Verification items for the finished model (mm, model axes). Round coordinates to 2 decimals unless told otherwise and drop trailing zeros. Order: outer loops, then holes, each group sorted by start corner. A loop starts at its lowest first (then second) coordinate and runs counter-clockwise, first axis right, second up.
```python
from build123d import *

# Parameters (mm, degrees)
BOSS_EXTRUDE1_DEPTH = 5
CUT_EXTRUDE1_DEPTH  = 1.5
CUT_EXTRUDE2_DEPTH  = 117.810049896
SKETCH1_11_R        = 5
CUT_EXTRUDE4_DEPTH  = 117.810049896


with BuildPart() as part:
    # Sketch1 → Boss-Extrude1 (new body)
    with BuildSketch(Plane(origin=(0, 0, 0), x_dir=(1, 0, 0), z_dir=(0, 1, 0))):
        Polygon((-89.9999746, -42.847712915), (-90.474893649, -60.847712915), (97.64978611, -63.907018624), (97.64978611, -43.907018893), align=None)
    extrude(amount=BOSS_EXTRUDE1_DEPTH)

    # Sketch1<7> → Cut-Extrude1 (cut)
    with BuildSketch(Plane(origin=(0, 0, 0), x_dir=(1, 0, 0), z_dir=(0, 1, 0))):
        with BuildLine():
            Line((-72.436927027, -45.130599461), (-72.436927027, -48.430599461))
            Line((-72.436927027, -48.430599461), (-87.431604768, -50.393286254))
            ThreePointArc((-87.431604768, -50.393286254), (-88.736927027, -51.880599461), (-87.431604768, -53.367912669))
            Line((-87.431604768, -53.367912669), (-72.436927027, -55.330599461))
            Line((-72.436927027, -55.330599461), (-72.436927027, -58.630599461))
            ThreePointArc((-72.436927027, -58.630599461), (-70.536927027, -60.530599461), (-68.636927027, -58.630599461))
            Line((-68.636927027, -58.630599461), (-68.636927027, -54.780599461))
            Line((-68.636927027, -54.780599461), (-55.641618403, -54.056431677))
            ThreePointArc((-55.641618403, -54.056431677), (-53.998192666, -52.22471247), (-55.641618403, -50.392993263))
            Line((-55.641618403, -50.392993263), (-68.636927027, -48.980599461))
            Line((-68.636927027, -48.980599461), (-68.636927027, -45.130599461))
            ThreePointArc((-68.636927027, -45.130599461), (-70.536927027, -43.230599461), (-72.436927027, -45.130599461))
        make_face()
    extrude(amount=CUT_EXTRUDE1_DEPTH, mode=Mode.SUBTRACT)

    # Sketch1<9> → Cut-Extrude2 (cut, through all)
    with BuildSketch(Plane(origin=(0, 0, 0), x_dir=(1, 0, 0), z_dir=(0, 1, 0))):
        with BuildLine():
            Line((-43.135065573, -46.112318891), (66.303161817, -46.73083337))
            ThreePointArc((66.303161817, -46.73083337), (73.096439635, -53.63791869), (66.153429754, -60.394424507))
            Line((66.153429754, -60.394424507), (-43.272048174, -58.614120743))
            ThreePointArc((-43.272048174, -58.614120743), (-49.421343824, -52.295091347), (-43.135065573, -46.112318891))
        make_face()
    extrude(amount=CUT_EXTRUDE2_DEPTH, mode=Mode.SUBTRACT)

    # Sketch1<11> → Cut-Extrude4 (cut, through all)
    with BuildSketch(Plane(origin=(0, 0, 0), x_dir=(1, 0, 0), z_dir=(0, 1, 0))):
        with Locations(Location((87.64978611, -53.797415464, 0), (0, 0, 270))):
            Circle(SKETCH1_11_R)
    extrude(amount=CUT_EXTRUDE4_DEPTH, mode=Mode.SUBTRACT)


solid = part.part
```
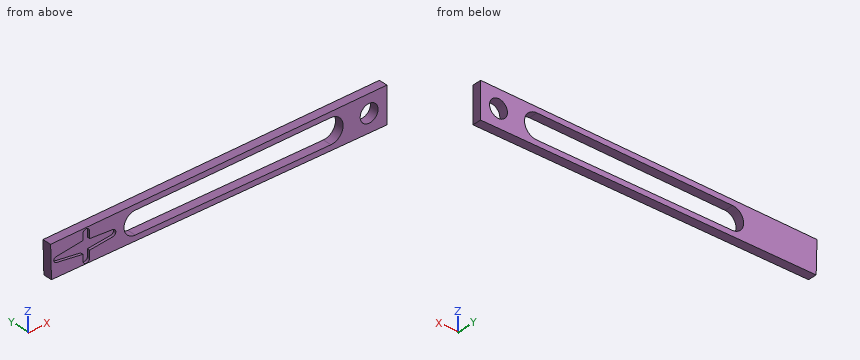
1) Scan lines: probe 1 along X at (y, z) = (4.7, 51); probe 2 along X at (y, z) = (2.5, 57); probe 3 along X at (y, z) = (1.45, 45). Record each from-to range of solid material in increasing order.
2) Sectioned sample at C-C on x = 39. Record the cut outline in (y, z), then the cut area to 3 significant figures.
3) Go/stop test with flat-tipped pins: pin 1 Ø1.2 at (y, z) = (1, 57.5) entering from -X; pin 2 Ø3 at (x, y) = (48.5, 2) entering from +Z; pin 3 Ø12 at (x, z) = (5, 47) entering from +Y; pin 4 Ø2 at (x, y) = (24, 3.5) entering from -Z. Record where each tip stops, or that it passes through.
4) Sectioned sample at A-A on x = 84.5. Record the cut outline in (y, z), then the cut area to 3 significant figures.
5) Sectioned sample at B-B on y = 3.9. Record the cut outline in (x, z).
Returned:
1. probe 1: x = -90.22 to -49.27, 72.6 to 83.51, 91.79 to 97.65
1. probe 2: x = -90.37 to -47.36, 72.17 to 83.81, 91.49 to 97.65
1. probe 3: x = -90.06 to -72.43, -68.64 to 97.65
2. outline: (0, 43.58) - (5, 43.58) - (5, 46.58) - (0, 46.58) - close; (0, 59.95) - (5, 59.95) - (5, 62.95) - (0, 62.95) - close
2. area: 30.0 mm2
3. pin 1: stops at x = -90.4
3. pin 2: stops at z = 63.13
3. pin 3: stops at y = 5
3. pin 4: stops at z = 43.49
4. outline: (0, 43.83) - (5, 43.83) - (5, 49.91) - (0, 49.91) - close; (0, 57.68) - (5, 57.68) - (5, 63.69) - (0, 63.69) - close
4. area: 60.5 mm2
5. outline: (-90.47, 60.85) - (-90, 42.85) - (97.65, 43.91) - (97.65, 63.91) - close; hole (-43.27, 58.61) arc R6.25 ccw to (-43.14, 46.11) - (66.3, 46.73) arc R6.83 ccw (long way) to (66.15, 60.39) - close; hole circle Ø10 at (87.65, 53.8)
